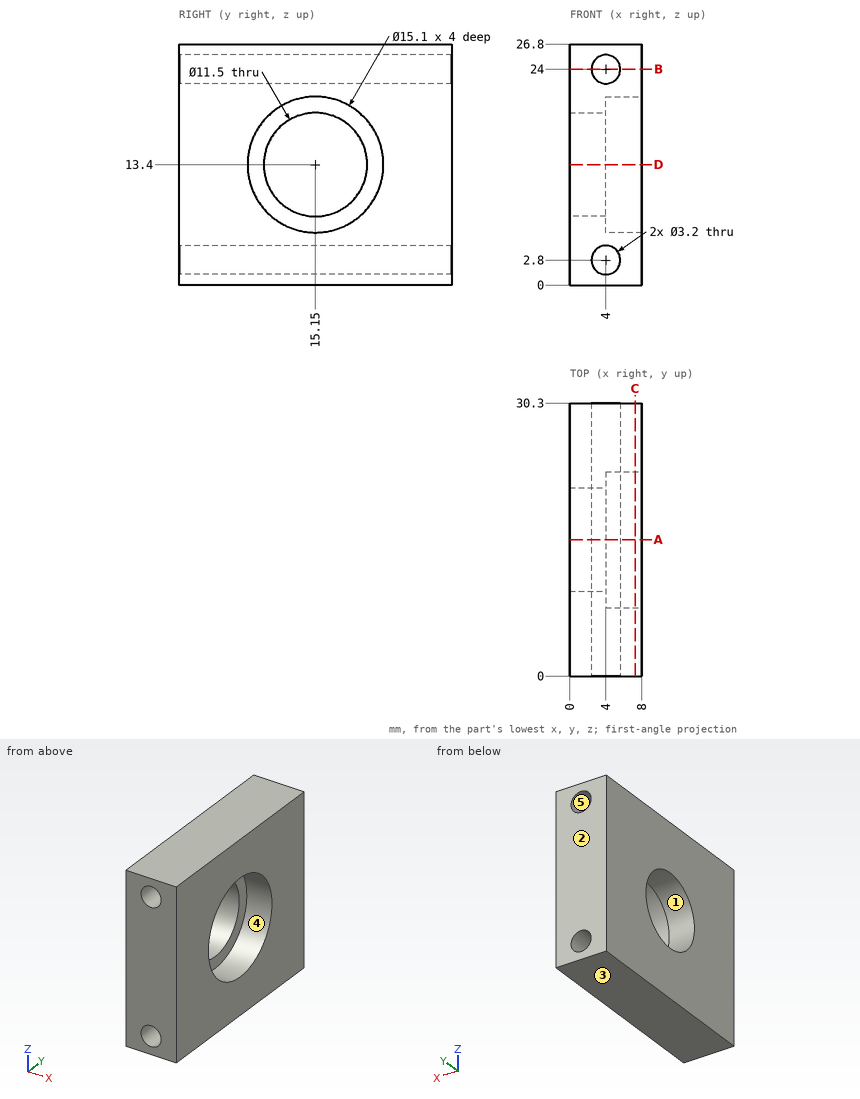
Answer from the drawing. Dimensions are ordinates in mm from the lowest x, y and z of the part. A direction names the side the tool comes from. Give positions to 0.01 mm unless a question says otherwise; leave off trailing zeros. Loops run counter-clockwise (first coordinate to the right, second up) from the corner with the lowest first, then second, coordinate; pieces in that order, holes last. Notation, with made-up numbers: (-17, 31.5) -> (34, 31.5) arc R24 ccw to (34, 64.5) -> close; hole circle Ø4 at (45, -39). An arc over 180 degrees is marked (long way). One line per question, with ' | ' between items. Start each with the question number.
1) Determine the mould class of the marked faces 1, 2 and 3 for opening direction Z: +Z half, -Z half, draft (parallel to the pull), parting line (faces both ways), or undercut.
2) Straight lines are drawn through the part: L1, parallel to X at y = 15, z = 2.8; L2, parallel to Y at x = 1.4, z = 13.4; L3, parallel to Y at x = 5.1, z = 13.4. For each, find the intervals that lie inside material, in ascending order.
3) Section B-B, the plane z = 24 is taken. Determine the outline of the cut face in (x, y), then the cut area to 3 significant figures.
4) For the marked faces 4 and 5, determine the directions among +Z, -Z, +X, -X, +Y, -Y from which every point of the face is accessible in a straight line to the end or side of a thin tool.
5) Section D-D, the plane z = 13.4 is taken. Determine the outline of the cut face in (x, y), then the cut area to 3 significant figures.
6) Section A-A, the plane y = 15.15 is taken. Determine the outline of the cut face in (x, z).
7) Section C-C, the plane x = 7.25 is taken. Determine the outline of the cut face in (y, z), then the cut area to 3 significant figures.
8) Each of these flat-tipped pins is pushed along its axis until it touches: pin 1 (15 mm diameter, centred on y = 15.15, z = 13.4, fed in from +X); pin 2 (3.5 mm diameter, centred on x = 4, z = 2.8, fed in from -Y); pin 3 (9 mm diameter, centred on y = 15.15, z = 13.4, fed in from -X). Where does it stop, or does it pass through?
Resolved:
1) face 1: undercut | face 2: draft | face 3: -Z half
2) L1: 0 to 2.4, 5.6 to 8 | L2: 0 to 9.4, 20.9 to 30.3 | L3: 0 to 7.6, 22.7 to 30.3
3) outline: (0, 0) -> (2.4, 0) -> (2.4, 30.3) -> (0, 30.3) -> close; (5.6, 0) -> (8, 0) -> (8, 30.3) -> (5.6, 30.3) -> close | area: 145 mm2
4) face 4: +X | face 5: +Y, -Y
5) outline: (0, 0) -> (8, 0) -> (8, 7.6) -> (4, 7.6) -> (4, 9.4) -> (0, 9.4) -> close; (0, 20.9) -> (4, 20.9) -> (4, 22.7) -> (8, 22.7) -> (8, 30.3) -> (0, 30.3) -> close | area: 136 mm2
6) outline: (0, 0) -> (8, 0) -> (8, 5.85) -> (4, 5.85) -> (4, 7.65) -> (0, 7.65) -> close; (0, 19.15) -> (4, 19.15) -> (4, 20.95) -> (8, 20.95) -> (8, 26.8) -> (0, 26.8) -> close; hole circle Ø3.2 at (4, 2.8); hole circle Ø3.2 at (4, 24)
7) outline: (0, 0) -> (30.3, 0) -> (30.3, 26.8) -> (0, 26.8) -> close; hole circle Ø15.1 at (15.15, 13.4) | area: 633 mm2
8) pin 1: x = 4 | pin 2: y = 0 | pin 3: through
